```python
from build123d import *

# Parameters (mm, degrees)
OTHER_START         = 7.189240539
OTHER_2_OUTLINE_W   = 16
OTHER_2_OUTLINE_H   = 16
OTHER_2_DEPTH       = 1.9877561
SKETCH_20_R         = 2.8
EXTRUDE_2_DEPTH     = 6.5
SKETCH_22_R         = 4
CUT_EXTRUDE_2_DEPTH = 9
CUT_EXTRUDE_3_DEPTH = 0.5


# Read off the part's stored shape, not the designer's step: 相交2
with BuildPart() as part:
    # 草图4 → Loft 1 section 0
    with BuildSketch(Plane(origin=(0, 8.2, 0), x_dir=(1, 0, 0), z_dir=(0, 1, 0))):
        with BuildLine():
            Line((-5.6, 6.8), (5.6, 6.8))
            Line((5.6, 6.8), (5.6, -5.7))
            Line((5.6, -5.7), (-5.6, -5.7))
            Line((-5.6, -5.7), (-5.6, 6.8))
        make_face()
    # 草图1 → Loft 1 section 1
    with BuildSketch(Plane(origin=(0, 0, 0), x_dir=(1, 0, 0), z_dir=(0, 1, 0))):
        with BuildLine():
            Line((-8.95, -8.9), (8.95, -8.9))
            Line((8.95, -8.9), (8.95, 8.9))
            Line((8.95, 8.9), (-8.95, 8.9))
            Line((-8.95, 8.9), (-8.95, -8.9))
        make_face()
    loft()

    # 相交2 outline → 相交2 (cut)
    with BuildSketch(Plane(origin=(0, 0, 0), x_dir=(1, 0, 0), z_dir=(0, 0.9872752829851917, -0.15902048800865198)).offset(OTHER_START)):
        Rectangle(OTHER_2_OUTLINE_W, OTHER_2_OUTLINE_H)
    extrude(amount=OTHER_2_DEPTH, mode=Mode.SUBTRACT)

    # 草图19 → Loft 1 2 section 0
    with BuildSketch(Plane(origin=(0, 6.132664073, -0.987788564), x_dir=(1, 0, 0), z_dir=(0, 0.9872752829851916, -0.15902048800865207))):
        with BuildLine():
            Line((-4.985089723, 5.299749211), (4.985089723, 5.299749211))
            Line((4.985089723, 5.299749211), (4.287230721, -5.442213697))
            Line((4.287230721, -5.442213697), (-4.287230721, -5.442213697))
            Line((-4.287230721, -5.442213697), (-4.985089723, 5.299749211))
        make_face()
    # 草图8 → Loft 1 2 section 1
    with BuildSketch(Plane.XZ):
        with BuildLine():
            Line((-7.15, 7.2), (7.15, 7.2))
            Line((7.15, 7.2), (7.15, -7.5))
            Line((7.15, -7.5), (-7.15, -7.5))
            Line((-7.15, -7.5), (-7.15, 7.2))
        make_face()
    loft(mode=Mode.SUBTRACT)

    # 草图20 → 凸台-拉伸2 (add)
    with BuildSketch(Plane.XZ):
        with Locations(Location((0, 0, 0), (0, 0, 270))):
            Circle(SKETCH_20_R)
        Polygon((-2.2, 0.8), (-0.8, 0.8), (-0.8, 2.2), (0.8, 2.2), (0.8, 0.8), (2.2, 0.8), (2.2, -0.8), (0.8, -0.8), (0.8, -2.2), (-0.8, -2.2), (-0.8, -0.8), (-2.2, -0.8), align=None, mode=Mode.SUBTRACT)
    extrude(amount=-EXTRUDE_2_DEPTH)

    # 草图22 → 切除-拉伸2 (cut)
    with BuildSketch(Plane.XZ):
        with Locations((-7, 9)):
            Circle(SKETCH_22_R)
    extrude(amount=-CUT_EXTRUDE_2_DEPTH, mode=Mode.SUBTRACT)

    # 草图23 → 切除-拉伸3 (cut)
    with BuildSketch(Plane(origin=(0, 7.097759487, -1.143236539), x_dir=(1, 0, 0), z_dir=(0, 0.9872752829851916, -0.15902048800865207))):
        Polygon((-4.255442902, 4.374408411), (-3.941340338, 4.374408411), (-3.941340338, 2.938510975), (-2.146468543, 2.938510975), (-2.146468543, 4.374408411), (-1.832365979, 4.374408411), (-1.832365979, 0.874408411), (-2.146468543, 0.874408411), (-2.146468543, 2.579536616), (-3.941340338, 2.579536616), (-3.941340338, 0.874408411), (-4.255442902, 0.874408411), align=None)
    extrude(amount=-CUT_EXTRUDE_3_DEPTH, mode=Mode.SUBTRACT)


solid = part.part
```
Check sheet for the modelled part. Datum: model origin and axes. Units: mm. A direction names the side the tool comes from. Round coordinates to 2 decimals unless told otherwise and drop trailing zeros. Answer as a JSON object with one key per item and string values. Group by question number.
Q1. Set-up check for faces 3 (the face through (0.8, 3, 2)), 4 (the face through (0, 6.5, 2.4)), 5 (the face through (-1, 0, -1)): record each of +Z, -Z, +X, -X, +Y, -Y from which the full face is reachable in a straight line by a thin tool's end or side.
Q2. Sectioned sample at A-A, the plane y = 4.25. Count the separate pieces of the cut face and the enclosed holes in it, plus the area to 3 significant figures.
Q3. Gauge pin test, flat ends, axial feed: P1, Ø4, axis at y = 1, z = 6, coming from the -X side; P2, Ø1.2, axis at x = 0.5, z = 2.5, coming from the +Y side; P3, Ø1, axis at y = 5, z = -2.5, coming from the +X side; P4, Ø1.5, axis at x = 7, z = 3.5, coming from the +Y side. Record the tip position at first contact, or that the pin passes through.
Q4. Mould release check, pull along X, two halves, no side actions. Record for faces 1 (the face through (8, 0, -1)), 2 (the face through (2.2, 3, 0)): released by +X, released by -X, zero draft, split by the parting line, or undercut.
Q5. Scan lines: line 1 along X through (y, z) = (0.5, 1); line 2 along X through (y, z) = (2.25, 2); line 3 along Z through (x, y) = (1, 3). Record each from-to range of solid material in increasing order. Write a range as [from, to].
Solution:
{
 "1": {"face 3": "-Y", "face 4": "none", "face 5": "+Z, -Z, +X, -X, -Y"},
 "2": {"separate pieces": "2", "enclosed holes": "1", "area": "94.6 mm²"},
 "3": {"P1": "stops at x = -8.95", "P2": "stops at y = 7.78", "P3": "stops at x = 7.11", "P4": "stops at y = 6.61"},
 "4": {"face 1": "zero draft", "face 2": "undercut"},
 "5": {"line 1": "x = [-8.75, -6.95], [-2.62, -0.8], [0.8, 2.62], [6.95, 8.75]", "line 2": "x = [-8.03, -6.23], [-1.96, -0.8], [0.8, 1.96], [6.23, 8.03]", "line 3": "z = [-8.13, -6.77], [-2.62, -0.8], [0.8, 2.62], [5.99, 7.73]"}
}
